Check sheet for the modelled part. Datum: model origin and axes. Units: mm. A direction names the side the tool comes from. Round coordinates to 2 decimals unless told otherwise and drop trailing zeros. Write each loop counter-clockwise with the first axis right and the second up, starting at its lowest first coordinate (ties: lowest second). Pieces come first, ordered by that corner, then holes. Notation, with made-up numbers: M 62.5,14.5 L 81.5,14.5 A21 ccw 81.5,31.5 Z; hole C 24,30.25 d3. An arc over 180 degrees is marked long. One line per item, written item: value.
from build123d import *

# Parameters (mm, degrees)
SKETCH1_W                  = 17.8
SKETCH1_H                  = 30
SKETCH1_R                  = 1
SKETCH1_R_2                = 2.5
BOSS_EXTRUDE1_DEPTH        = 2.5
SKETCH2_W                  = 9
SKETCH2_H                  = 6
SKETCH2_W_2                = 5
SKETCH2_H_2                = 5.830943002
CUT_EXTRUDE1_DEPTH         = 20.350968968
CHAMFER1_SIZE              = 2
FILLET1_R                  = 1
BOSS_EXTRUDE2_DEPTH        = 1
SKETCH4_W                  = 12
SKETCH4_H                  = 18.95
BOSS_EXTRUDE3_DEPTH        = 4
BOSS_EXTRUDE4_DEPTH        = 37.9
SKETCH6_W                  = 12.770133269
SKETCH6_H                  = 37.9
BOSS_EXTRUDE5_DEPTH        = 11.41
F_3_0_MM_DOWEL_HOLES1_D    = 3
F_4_2_4_2_DIAMETER_HOLE1_D = 4.2


with BuildPart() as part:
    # Sketch1 → Boss-Extrude1 (new body)
    with BuildSketch(Plane(origin=(0, 0, 0), x_dir=(1, 0, 0), z_dir=(0, 1, 0))):
        with Locations((0, -2)):
            Rectangle(SKETCH1_W, SKETCH1_H)
        with Locations(Location((-6.9, 0, 0), (0, 0, 270))):
            Circle(SKETCH1_R, mode=Mode.SUBTRACT)
        with Locations(Location((6.9, 0, 0), (0, 0, 270))):
            Circle(SKETCH1_R, mode=Mode.SUBTRACT)
        with Locations(Location((0, 5.3, 0), (0, 0, 270))):
            Circle(SKETCH1_R_2, mode=Mode.SUBTRACT)
    extrude(amount=BOSS_EXTRUDE1_DEPTH)

    # Sketch2 → Cut-Extrude1 (cut, through all)
    with BuildSketch(Plane(origin=(0, 2.5, 0), x_dir=(1, 0, 0), z_dir=(0, 1, 0))):
        with Locations((0, -6.5)):
            Rectangle(SKETCH2_W, SKETCH2_H)
        with Locations((0, -12.415471501)):
            Rectangle(SKETCH2_W_2, SKETCH2_H_2)
    extrude(amount=-CUT_EXTRUDE1_DEPTH, mode=Mode.SUBTRACT)

    # Chamfer1
    chamfer1_edges = [part.edges().sort_by_distance(p)[0] for p in [
        (2.5, 1.25, 9.5),
        (-2.5, 1.25, 9.5),
    ]]
    chamfer(chamfer1_edges, length=CHAMFER1_SIZE - 0.0001)  # a hair under: the kernel refuses the full size

    # Fillet1
    fillet1_edges = [part.edges().sort_by_distance(p)[0] for p in [
        (4.5, 1.25, 3.5),
        (2.5, 1.25, 15.330943002),
        (-2.5, 1.25, 15.330943002),
        (-4.5, 1.25, 3.5),
    ]]
    fillet(fillet1_edges, radius=FILLET1_R)

    # Sketch3 → Boss-Extrude2 (add)
    with BuildSketch(Plane(origin=(0, 2.5, 0), x_dir=(1, 0, 0), z_dir=(0, 1, 0))):
        with BuildLine():
            Line((8.84, 8.16), (6.959390471, 8.16))
            ThreePointArc((6.959390471, 8.16), (6.042112051, 10.284532913), (3.900010938, 11.159999998))
            Line((3.900010938, 11.159999998), (-3.900010938, 11.159999998))
            ThreePointArc((-3.900010938, 11.159999998), (-6.04211205, 10.284532912), (-6.959390471, 8.16))
            Line((-6.959390471, 8.16), (-8.84, 8.16))
            Line((-8.84, 8.16), (-8.84, 12.94))
            Line((-8.84, 12.94), (8.84, 12.94))
            Line((8.84, 12.94), (8.84, 8.16))
        make_face()
    extrude(amount=BOSS_EXTRUDE2_DEPTH)

    # Sketch4 → Boss-Extrude3 (add)
    with BuildSketch(Plane.ZY.offset(8.9)):
        with Locations((-7, 9.475)):
            Rectangle(SKETCH4_W, SKETCH4_H)
    extrude(amount=BOSS_EXTRUDE3_DEPTH)

    # Mirror2: part across plane


with BuildPart() as part_1:
    add(part.part)
    add(part.part.mirror(Plane.ZX.offset(18.95)))

    # Sketch5 → Boss-Extrude4 (add)
    with BuildSketch(Plane(origin=(0, 37.9, 0), x_dir=(1, 0, 0), z_dir=(0, 1, 0))):
        Polygon((-12.9, 1), (-17.267642811, 13), (-12.9, 13), align=None)
    extrude(amount=-BOSS_EXTRUDE4_DEPTH)

    # Sketch6 → Boss-Extrude5 (add)
    with BuildSketch(Plane(origin=(-11.069592853, 0, 4.029002304), x_dir=(0.3420201433256634, 0, 0.9396926207859103), z_dir=(-0.9396926207859103, 0, 0.3420201433256634))):
        with Locations((-11.736819105, 18.95)):
            Rectangle(SKETCH6_W, SKETCH6_H)
    extrude(amount=BOSS_EXTRUDE5_DEPTH)

    # Ø3.0 mm Dowel Holes1 (through all)
    with Locations(Plane(origin=(-23.72675034, 0, 2.614356121), x_dir=(-0.34202014332566333, 0, -0.9396926207859103), z_dir=(-0.9396926207859104, 0, 0.3420201433256634))):
        with Locations((5.693417073, -6.95), (5.693417073, -30.95)):
            Hole(F_3_0_MM_DOWEL_HOLES1_D / 2)

    # Ø4.2 (4.2) Diameter Hole1 (through all)
    with Locations(Plane(origin=(-21.791485656, 0, 7.931452139), x_dir=(0.34202014332566333, 0, 0.9396926207859103), z_dir=(-0.9396926207859104, 0, 0.3420201433256634))):
        with Locations((-11.35175247, 13.95), (-11.35175247, 23.95)):
            Hole(F_4_2_4_2_DIAMETER_HOLE1_D / 2)


solid = part_1.part
Q1. Sectioned sample at D-D on z = 9. Enter the section's corners in (x, y), and give its area (3 significant figures).
Completed:
outline: M -8.9,0 L -4.5,0 L -4.5,2.5 L -8.9,2.5 Z; M -8.9,35.4 L -4.5,35.4 L -4.5,37.9 L -8.9,37.9 Z; M 4.5,0 L 8.9,0 L 8.9,2.5 L 4.5,2.5 Z; M 4.5,35.4 L 8.9,35.4 L 8.9,37.9 L 4.5,37.9 Z
area: 44.0 mm^2
Q2. Access from +Z, -Z, +X, -X, +Y, -Y to the whole of each face (thin tool, end or side, straight path). Record for faces 3 (the flat face through (-11, 19, -1)), 4 (the flat face through (-4.5, 37, 7)), 5 (the flat face through (0, 35, -12.94)), 6 (the flat face through (8.84, 35, -11)), 7 (the cylindrical face through (6.066, 2.993, -10.261)).
Completed:
face 3: +Z, +Y, -Y
face 4: +Y, -Y
face 5: -Z, +X
face 6: +Z, -Z, +X
face 7: +Z
Q3. Sectioned sample at C-C on y = 13. Enter the section's corners in (x, z).
Completed:
outline: M -27.99,-9.1 L -17.27,-13 L -8.9,-13 L -8.9,-10.83 L -26.31,-4.5 Z; M -25.03,-0.98 L -8.9,-6.85 L -8.9,-1 L -12.9,-1 L -23.62,2.9 Z
Q4. Scan lines: line 1 (Y direction, x = -6, z = 6); line 2 (Z direction, x = -12, y = 29); line 3 (X direction, y = 36.05, z = -5.3). Record each from-to range of solid material in increasing order. Write a range as [from, to].
Completed:
line 1: [0, 2.5], [35.4, 37.9]
line 2: [-13, -1]
line 3: [-26.61, -2.5], [2.5, 8.9]
Q5. Sectioned sample at A-A on z = 13. Enter the section's corners in (x, y).
Completed:
outline: M -8.9,0 L -2.5,0 L -2.5,2.5 L -8.9,2.5 Z; M -8.9,35.4 L -2.5,35.4 L -2.5,37.9 L -8.9,37.9 Z; M 2.5,0 L 8.9,0 L 8.9,2.5 L 2.5,2.5 Z; M 2.5,35.4 L 8.9,35.4 L 8.9,37.9 L 2.5,37.9 Z
Q6. Depth check by flat-ended pin: P1, Ø1.1, axis at y = 35, z = -10.5, coming from the +X side; P2, Ø8, axis at x = -21.5, y = 17.5, coming from the -Z side; P3, Ø10, axis at x = -18, y = 26.5, coming from the +Z side; P4, Ø0.8, axis at y = 1.5, z = 5, coming from the -X side. Enter the tip coordinate at first touch or a pass-through.
Completed:
P1: x = 8.9
P2: z = -12.92
P3: z = 2.68
P4: x = -8.9
Q7. Draft check along Y on faces 1 (the flat face through (-18.186, 18.685, 0.924)), 2 (the cylindrical face through (-6.018, 34.907, -10.308)). Enter one of: pulls with the +Y half, pulls with the -Y half, needs draft (parallel to the pull), parting line crosses it, or undercut.
Completed:
face 1: needs draft
face 2: undercut
Q8. Sectioned sample at B-B on x = 0. State how many separate pieces and enclosed holes the cut face has, and give its area (3 significant figures).
Completed:
separate pieces: 6
enclosed holes: 0
area: 69.4 mm^2
